Source: CAD feature listing. Evaluate the final solid. Frame: model axes, mm. A direction names the side the tool comes from. Give positions to 0.01 mm unless a question says otherwise; leave off trailing zeros. Loops run counter-clockwise (first coordinate to the right, second up) from the corner with the lowest first, then second, coordinate; pieces in that order, holes last. Notation, with made-up numbers: (28, 27.25) - (81, 27.25) arc R28 ccw to (81, 57.25) - close; hole circle Ø5 at (77, 3). An arc over 180 degrees is marked (long way). Write each question's results on one line, items separated by ' | '. Start each with the question number.
(1) Reachability of faces 1 (the flat face through (-43.894, 69.197, 69.368)), 2 (the cylindrical face through (-74.153, 3.402, 40.56)) from +Z, -Z, +X, -X, +Y, -Y: full face, straight path, thin tool, end or side. Return the list, or none.
(2) Cut plane A-A on z = 13.5. Return the cut outline in (x, y).
(3) Pull-direction query (Z, two-part tool) for faces 3 (the cylindrical face through (-78.95, 4.01, 9.11)), 4 (the cylindrical face through (-60.451, 35.293, 39.44)), 5 (the flat face through (-62, 34, 80)), 6 (the flat face through (-82.95, 1.55, 8.48)); classes: pulls with the +Z half, pulls with the -Z half, needs draft (parallel to the pull), parting line crosses it, or undercut.
(4) Cut plane C-C on y = 20.5. Return the cut outline in (x, z), then the cut area to 3 significant figures.
(5) Contact query for flat-ended pins moving along their axis: pin 1 (4 mm diameter, centred on x = -52.5, y = 59.5, fed in from -Z); pin 2 (12 mm diameter, centred on y = 11.5, z = 71.5, fed in from +X); pin 3 (6 mm diameter, centred on y = 37.5, z = 34, fed in from -X); pin 4 (1 mm diameter, centred on x = -76.5, z = 25, fed in from -Y). Output: stop coordinate, or through.
(6) Cut plane B-B on x = -59. Return the cut outline in (y, z).
(7) Material intervals for line 1 along Y through (x, z) = (-50, 44.5); line 2 along Y through (x, z) = (-80.5, 72); line 3 along X through (y, z) = (44.5, 74.5), sorted ascending. Write a range as [from, to].
from build123d import *

# Parameters (mm, degrees)
BOSS_EXTRUDE1_DEPTH       = 80
FILLET1_R                 = 15
FILLET2_R                 = 15
SKETCH3_R                 = 2.5
CUT_EXTRUDE1_DEPTH        = 10
SKETCH3_2_R               = 2.5
BOSS_EXTRUDE2_DEPTH       = 1
SKETCH5_R                 = 1.5
CUT_EXTRUDE2_DEPTH        = 1
LPATTERN1_COUNT           = 2
LPATTERN1_PITCH           = 62
LPATTERN2_COUNT           = 2
LPATTERN2_PITCH           = 77
LPATTERN2_COPY_1_SKETCH_R = 2.5
LPATTERN2_COPY_1_DEPTH    = 10
LPATTERN2_COPY_2_SKETCH_R = 2.5
LPATTERN2_COPY_2_DEPTH    = 1
LPATTERN2_COPY_3_SKETCH_R = 1.5
LPATTERN2_COPY_3_DEPTH    = 1


with BuildPart() as part:
    # Sketch2 → Boss-Extrude1 (new body)
    with BuildSketch(Plane.XY):
        with BuildLine():
            Line((-70, 0), (-85, 0))
            Line((-85, 0), (-42.5, 73.612159322))
            Line((-42.5, 73.612159322), (-35, 60.621778265))
            ThreePointArc((-35, 60.621778265), (-60.621778265, 35), (-70, 0))
        make_face()
    extrude(amount=BOSS_EXTRUDE1_DEPTH)

    # Fillet1
    fillet1_edges = [part.edges().sort_by_distance(p)[0] for p in [
        (-70, 0, 40),
    ]]
    fillet(fillet1_edges, radius=FILLET1_R)

    # Fillet2
    fillet2_edges = [part.edges().sort_by_distance(p)[0] for p in [
        (-35, 60.621778265, 40),
    ]]
    fillet(fillet2_edges, radius=FILLET2_R)

    # Sketch3 → Cut-Extrude1 (cut)
    with BuildSketch(Plane(origin=(-63.75, 36.806079661, 0), x_dir=(0, 0, 1), z_dir=(-0.866025403784438, 0.5000000000000011, 0))):
        with Locations(Location((9, 38.5, 0), (0, 0, 270))):
            Circle(SKETCH3_R)
    cut_extrude1 = extrude(amount=-CUT_EXTRUDE1_DEPTH, mode=Mode.SUBTRACT)

    # Sketch3_2 → Boss-Extrude2 (add)
    with BuildSketch(Plane(origin=(-63.75, 36.806079661, 0), x_dir=(0, 0, 1), z_dir=(-0.866025403784438, 0.5000000000000011, 0))):
        with Locations(Location((9, 38.5, 0), (0, 0, 270))):
            Circle(SKETCH3_2_R)
    boss_extrude2 = extrude(amount=-BOSS_EXTRUDE2_DEPTH)

    # Sketch5 → Cut-Extrude2 (cut)
    with BuildSketch(Plane(origin=(-63.75, 36.806079661, 0), x_dir=(0, 0, 1), z_dir=(-0.866025403784438, 0.5000000000000011, 0))):
        with Locations(Location((9, 38.5, 0), (0, 0, 270))):
            Circle(SKETCH5_R)
    cut_extrude2 = extrude(amount=-CUT_EXTRUDE2_DEPTH, mode=Mode.SUBTRACT)

    # LPattern1: Cut-Extrude1, Boss-Extrude2, Cut-Extrude2 ×2
    with Locations(*[(0, 0, i * LPATTERN1_PITCH) for i in range(1, LPATTERN1_COUNT)]):
        add(cut_extrude1, mode=Mode.SUBTRACT)
        add(boss_extrude2)
        add(cut_extrude2, mode=Mode.SUBTRACT)

    # LPattern2: Cut-Extrude1, Boss-Extrude2, Cut-Extrude2 ×2
    with Locations(*[Vector(-0.5000000000000009, -0.8660254037844383, 0) * (i * LPATTERN2_PITCH) for i in range(1, LPATTERN2_COUNT)]):
        add(cut_extrude1, mode=Mode.SUBTRACT)
        add(boss_extrude2)
        add(cut_extrude2, mode=Mode.SUBTRACT)

    # LPattern2 copy 1 sketch → LPattern2 copy 1 (cut)
    with BuildSketch(Plane(origin=(-102.25, -29.877876431, 62), x_dir=(0, 0, 1), z_dir=(-0.866025403784438, 0.5000000000000011, 0))):
        with Locations(Location((9, 38.5, 0), (0, 0, 270))):
            Circle(LPATTERN2_COPY_1_SKETCH_R)
    extrude(amount=-LPATTERN2_COPY_1_DEPTH, mode=Mode.SUBTRACT)

    # LPattern2 copy 2 sketch → LPattern2 copy 2 (add)
    with BuildSketch(Plane(origin=(-102.25, -29.877876431, 62), x_dir=(0, 0, 1), z_dir=(-0.866025403784438, 0.5000000000000011, 0))):
        with Locations(Location((9, 38.5, 0), (0, 0, 270))):
            Circle(LPATTERN2_COPY_2_SKETCH_R)
    extrude(amount=-LPATTERN2_COPY_2_DEPTH)

    # LPattern2 copy 3 sketch → LPattern2 copy 3 (cut)
    with BuildSketch(Plane(origin=(-102.25, -29.877876431, 62), x_dir=(0, 0, 1), z_dir=(-0.866025403784438, 0.5000000000000011, 0))):
        with Locations(Location((9, 38.5, 0), (0, 0, 270))):
            Circle(LPATTERN2_COPY_3_SKETCH_R)
    extrude(amount=-LPATTERN2_COPY_3_DEPTH, mode=Mode.SUBTRACT)


solid = part.part
Ans:
1) face 1: none | face 2: +Z, -Z, +X, -Y
2) outline: (-85, 0) - (-83.67, 0) arc R15 ccw to (-68.9, 12.35) arc R70 cw to (-45.15, 53.49) arc R15 ccw to (-41.83, 72.46) - (-42.5, 73.61) - close
3) face 3: undercut | face 4: needs draft | face 5: pulls with the +Z half | face 6: undercut
4) outline: (-73.16, 0) - (-66.93, 0) - (-66.93, 80) - (-73.16, 80) - close | area: 499 mm^2
5) pin 1: z = 0 | pin 2: x = -67.78 | pin 3: x = -65.08 | pin 4: y = 1.56
6) outline: (37.67, 0) - (45.03, 0) - (45.03, 80) - (37.67, 80) - close
7) line 1: [48.99, 60.62] | line 2: [4.67, 7.79] | line 3: [-59.31, -54.03]
